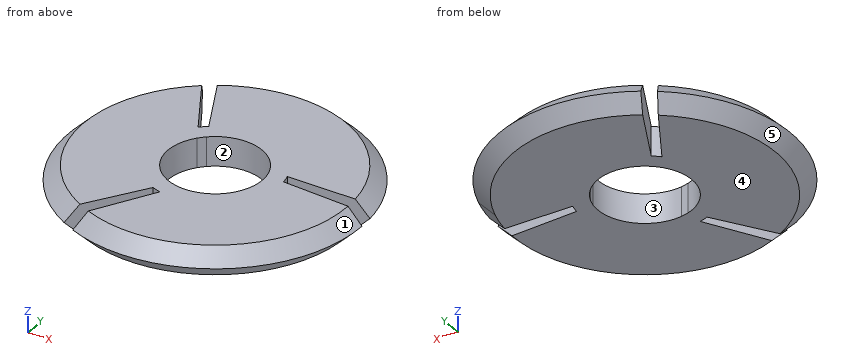
from build123d import *

# Parameters (mm, degrees)
F1_DEPTH     = 7
F2_T2_ANGLE  = 147.8228871573
F2_T4_ANGLE  = 147.8228871573
F2_T6_ANGLE  = 147.8228871573
F2_T8_ANGLE  = 147.8228871573
F2_T10_ANGLE = 147.8228871573
F2_T12_ANGLE = 147.8228871573


# Not quite as in the source:
# - a fillet or chamfer that OpenCascade refuses, or shapes differently, is made with other operations: its cross-section is extruded or revolved along the edge and cut away or added


with BuildPart() as f1:
    # F0 (on Top) → F1 (new body)
    with BuildSketch(Plane.XY):
        with BuildLine():
            Line((-28.4060324401, -36.6326823344), (-16.7057452382, -20.1458706432))
            ThreePointArc((-16.7057452382, -20.1458706432), (-25.4681782111, -8.7912963767), (-20.97968548, 4.8307453711))
            Line((-20.97968548, 4.8307453711), (-30.6144689612, 22.7902857677))
            ThreePointArc((-30.6144689612, 22.7902857677), (-45.7201890255, -7.5236357069), (-28.4060324401, -36.6326823344))
        make_face()
        with BuildLine():
            ThreePointArc((-19.29435824, 6.2304415143), (-5.0797919896, 8.1416439346), (4.4729958499, -2.5565256692))
            Line((4.4729958499, -2.5565256692), (24.8438058142, -3.1923286128))
            ThreePointArc((24.8438058142, -3.1923286128), (6.144039761, 25.0465694426), (-27.722212391, 24.6065933083))
            Line((-27.722212391, 24.6065933083), (-19.29435824, 6.2304415143))
        make_face()
        with BuildLine():
            ThreePointArc((4.9156669829, -6.2104463577), (-1.1968722093, -18.4456132191), (-14.6509092006, -20.9055587751))
            Line((-14.6509092006, -20.9055587751), (-25.3869356838, -38.229296228))
            ThreePointArc((-25.3869356838, -38.229296228), (8.4185504337, -36.154272809), (24.9706460004, -6.6052500471))
            Line((24.9706460004, -6.6052500471), (4.8425046474, -4.7159099443))
            ThreePointArc((4.8425046474, -4.7159099443), (4.8973654542, -5.4622833042), (4.9156669829, -6.2104463577))
        make_face()
        with BuildLine():
            Line((-16.7057452382, -20.1458706432), (-14.3009175091, -16.7572408399))
            ThreePointArc((-14.3009175091, -16.7572408399), (-21.2699622014, -9.0563128177), (-18.9622633915, 1.0702069463))
            Line((-18.9622633915, 1.0702069463), (-20.97968548, 4.8307453711))
            ThreePointArc((-20.97968548, 4.8307453711), (-25.4681782111, -8.7912963767), (-16.7057452382, -20.1458706432))
        make_face()
        with BuildLine():
            ThreePointArc((-17.5621326109, 2.4534847075), (-7.4084109648, 4.63839044), (0.2075629978, -2.4233952356))
            Line((0.2075629978, -2.4233952356), (4.4729958499, -2.5565256692))
            ThreePointArc((4.4729958499, -2.5565256692), (-5.0797919896, 8.1416439346), (-19.29435824, 6.2304415143))
            Line((-19.29435824, 6.2304415143), (-17.5621326109, 2.4534847075))
        make_face()
        with BuildLine():
            ThreePointArc((0.7054512892, -4.3275829408), (-2.4792256646, -14.2134166955), (-12.4028984371, -17.2781507839))
            Line((-12.4028984371, -17.2781507839), (-14.6509092006, -20.9055587751))
            ThreePointArc((-14.6509092006, -20.9055587751), (-1.1968722093, -18.4456132191), (4.9156669829, -6.2104463577))
            ThreePointArc((4.9156669829, -6.2104463577), (4.8973654542, -5.4622833042), (4.8425046474, -4.7159099443))
            Line((4.8425046474, -4.7159099443), (0.7054512892, -4.3275829408))
        make_face()
        with BuildLine():
            Line((-20.97968548, 4.8307453711), (-18.9622633915, 1.0702069463))
            ThreePointArc((-18.9622633915, 1.0702069463), (-18.2773306397, 1.7771628324), (-17.5621326109, 2.4534847075))
            Line((-17.5621326109, 2.4534847075), (-19.29435824, 6.2304415143))
            ThreePointArc((-19.29435824, 6.2304415143), (-20.1621039238, 5.5607939156), (-20.97968548, 4.8307453711))
        make_face()
        with BuildLine():
            ThreePointArc((0.2075629978, -2.4233952356), (0.4773383786, -3.3700423415), (0.7054512892, -4.3275829408))
            Line((0.7054512892, -4.3275829408), (4.8425046474, -4.7159099443))
            ThreePointArc((4.8425046474, -4.7159099443), (4.6964456573, -3.6295963387), (4.4729958499, -2.5565256692))
            Line((4.4729958499, -2.5565256692), (0.2075629978, -2.4233952356))
        make_face()
        with BuildLine():
            Line((-14.6509092006, -20.9055587751), (-12.4028984371, -17.2781507839))
            Line((-12.4028984371, -17.2781507839), (-14.3009175091, -16.7572408399))
            Line((-14.3009175091, -16.7572408399), (-16.7057452382, -20.1458706432))
            ThreePointArc((-16.7057452382, -20.1458706432), (-15.6919405642, -20.56253665), (-14.6509092006, -20.9055587751))
        make_face()
    extrude(amount=F1_DEPTH)

    # F2: chamfer of 4 on 6 edges, made by hand

    # F2_s1 → F2_t2 (revolve, cut)
    with BuildSketch(Plane(origin=(-11.2150452206, -3.6909975733, 0), x_dir=(0, 0, 1), z_dir=(0.9498795724, 0.3126160553, 0))):
        Polygon((3, -32.7063288851), (7, -28.7063288851), (7, -32.7063288851), align=None)
    revolve(axis=Axis((-10.3858662769, -6.2104463577, 7), (0, 0, 1)), revolution_arc=F2_T2_ANGLE, mode=Mode.SUBTRACT)

    # F2_s3 → F2_t4 (revolve, cut)
    with BuildSketch(Plane(origin=(-11.2150452206, -3.6909975733, 0), x_dir=(0, 0, 1), z_dir=(0.9498795724, 0.3126160553, 0))):
        Polygon((4, -32.7063288851), (0, -28.7063288851), (0, -32.7063288851), align=None)
    revolve(axis=Axis((-10.3858662769, -6.2104463577, 0), (0, 0, 1)), revolution_arc=F2_T4_ANGLE, mode=Mode.SUBTRACT)

    # F2_s5 → F2_t6 (revolve, cut)
    with BuildSketch(Plane(origin=(-2.6891726039, 2.4029660659, 0), x_dir=(0, 0, 1), z_dir=(-0.7456732317, 0.6663118126, 0))):
        Polygon((3, -46.9099054592), (7, -42.9099054592), (7, -46.9099054592), align=None)
    revolve(axis=Axis((-10.3858662769, -6.2104463577, 7), (0, 0, 1)), revolution_arc=F2_T6_ANGLE, mode=Mode.SUBTRACT)

    # F2_s7 → F2_t8 (revolve, cut)
    with BuildSketch(Plane(origin=(-2.6891726039, 2.4029660659, 0), x_dir=(0, 0, 1), z_dir=(-0.7456732317, 0.6663118126, 0))):
        Polygon((4, -46.9099054592), (0, -42.9099054592), (0, -46.9099054592), align=None)
    revolve(axis=Axis((-10.3858662769, -6.2104463577, 0), (0, 0, 1)), revolution_arc=F2_T8_ANGLE, mode=Mode.SUBTRACT)

    # F2_s9 → F2_t10 (revolve, cut)
    with BuildSketch(Plane(origin=(-1.6745815909, -8.0276380292, 0), x_dir=(0, 0, 1), z_dir=(-0.2042063407, -0.9789278678, 0))):
        Polygon((3, -26.4599150641), (7, -22.4599150641), (7, -26.4599150641), align=None)
    revolve(axis=Axis((-10.3858662769, -6.2104463577, 7), (0, 0, 1)), revolution_arc=F2_T10_ANGLE, mode=Mode.SUBTRACT)

    # F2_s11 → F2_t12 (revolve, cut)
    with BuildSketch(Plane(origin=(-1.6745815909, -8.0276380292, 0), x_dir=(0, 0, 1), z_dir=(-0.2042063407, -0.9789278678, 0))):
        Polygon((4, -26.4599150641), (0, -22.4599150641), (0, -26.4599150641), align=None)
    revolve(axis=Axis((-10.3858662769, -6.2104463577, 0), (0, 0, 1)), revolution_arc=F2_T12_ANGLE, mode=Mode.SUBTRACT)


solid = f1.part
Input: part model. Units: mm. Frame: model coordinates. Face numbers are marked on the shaded views. A direction names the side the tool comes from. Give positions to 0.01 mm unless a question says otherwise; leave off trailing zeros. Order: outer loops, then holes, each group sorted by start corner. A loop starts at its lowest first (then second) coordinate and runs counter-clockwise, first axis right, second up. Notation, with made-up numbers: (67, 59) -> (96, 59) arc R25 cw to (96, 81) -> close; hole circle Ø7 at (63, 77). An arc over 180 degrees is marked (long way). Use one line per item in the form item = value.
1) Section A-A, the plane z = 4.5. Return loops of the section in (x, y).
Response values:
outline = (-29.9, 21.46) arc R33.86 ccw to (-27.53, -35.41) -> (-16.71, -20.15) arc R15.3 ccw to (-14.65, -20.91) -> (-24.59, -36.95) arc R33.86 ccw to (23.47, -6.46) -> (4.84, -4.72) arc R15.3 ccw to (4.47, -2.56) -> (23.33, -3.15) arc R33.86 ccw to (-27.09, 23.24) -> (-19.29, 6.23) arc R15.3 ccw to (-20.98, 4.83) -> close; hole (-18.96, 1.07) arc R11.25 ccw to (-14.3, -16.76) -> (-12.4, -17.28) arc R11.25 ccw to (0.71, -4.33) arc R22.5 ccw to (0.21, -2.42) arc R11.25 ccw to (-17.56, 2.45) arc R22.5 ccw to start
2) Mould query, pull axis X, two halves, no side actions, for the marked faces 3, 4 and 5. Classes: pulls with the +X half, pulls with the -X half, needs draft (parallel to the pull), parting line crosses it, or undercut.
Response values:
face_3 = undercut
face_4 = needs draft
face_5 = pulls with the -X half
3) First-contact query: pin 1 Ø8 at (x, y) = (12.5, -12.5) entering from -Z; pin 2 Ø1.5 at (y, z) = (-20.5, 2.5) entering from -X; pin 3 Ø2 at (x, z) = (16.5, 3.5) entering from -Y. Flat tips, straight axial feed; report the tip coordinate or a pass-through.
Response values:
pin_1 = 0
pin_2 = -41.97
pin_3 = -29.56
4) Reachability of the marked faces 1 and 2 from +Z, -Z, +X, -X, +Y, -Y: full face, straight path, thin tool, end or side. Return the list, or none.
Response values:
face_1 = +Z, -Y
face_2 = +Z, -Z
5) Line query: probe 1 along Y at (x, z) = (-22.5, 6); probe 2 along X at (y, z) = (18.5, 1.5); probe 3 along Y at (x, z) = (-20.5, 5). Output: solid intervals per line, ascending.
Response values:
probe_1 = -36.22 to -33.57, -28.31 to 7.66, 13.22 to 23.8
probe_2 = -32.04 to -28.31, -24.92 to 11.27
probe_3 = -38 to -30.34, -25.49 to -11.14, -1.28 to 5.27, 8.86 to 25.58
